Could you check a few things on this model? Use its own coordinates, in mm. Face numbers are marked on the shaded views. A direction names the side the tool comes from. Round coordinates to 2 decimals unless told otherwise and drop trailing zeros. Write each loop counter-clockwise with the first axis right and the second up, starting at its lowest first coordinate (ties: lowest second). Pieces come first, ordered by that corner, then holes. Notation, with made-up numbers: (-16, -35.75) -> (33, -35.75) arc R28 ccw to (33, -9.75) -> close; hole circle Ø10 at (62, 5.25). An arc over 180 degrees is marked (long way). Answer as CSV lines item,"result". Start each with the question number.
Q1. Imagine slicing it at D-D on x = -1.75. Please give me the cut outline in (y, z).
Q2. Imagine slicing it at B-B on x = 0. Please give me the cut outline in (y, z), and give its area (3 significant figures).
Q3. Imagine slicing it at A-A on y = 0. Please give me the cut outline in (x, z), and give its area (3 significant figures).
Q4. For the marked faces 1, 2 and 3, which set-ups out of +Z, -Z, +X, -X, +Y, -Y let a thin tool reach every point of the face, with its end or its side?
Q5. If I drill on line 1 (X direction, y = 0.1, z = 13); line 2 (Z direction, x = 0, y = 0.1); line 3 (Y direction, x = -2, z = 5.25), over which ranges is the centre line in solid material (lowest first)? Write a range as [from, to].
Q6. Will these pins go through, and if not, where does the flat tip stop? pin 1 Ø1 at (x, y) = (3, -1.5) entering from +Z; pin 2 Ø1 at (x, z) = (-3.5, 11) entering from -Y; pin 3 Ø1.1 at (y, z) = (0, 5) entering from -X.
Q7. Imagine slicing it at C-C on z = 13. Please give me the cut outline in (x, y), and give its area (3 significant figures).
Autodesk Inventor part; units mm, degrees
ref_plane "YZ Plane" through (0, 0, 0) normal (1, 0, 0) x (0, 1, 0)
ref_plane "XZ Plane" through (0, 0, 0) normal (0, 1, 0) x (-1, 0, 0)
ref_plane "XY Plane" through (0, 0, 0) normal (0, 0, 1) x (1, 0, 0)
sketch "Skizze1" plane through (0, 0, 0) normal (0, 0, 1) x (1, 0, 0)
  circle A0 centre (0, 0) radius 6.5
  dimension "d11" = 13
extrude "Extrusion1" add sketch "Skizze1" along normal blind 1
sketch "Skizze2" plane through (0, 0, 0) normal (0, 1, 0) x (-1, 0, 0)
  line L0 (6.5, 1) -> (-6.5, 1)
  line L1 (3.5, 1) -> (-3.5, 1)
  line L2 (-3.5, 1) -> (-3.5, 16)
  line L3 (-3.5, 16) -> (3.5, 16)
  line L4 (3.5, 16) -> (3.5, 1)
  line L5 (0, -1) -> (0, 20)
  circle A0 centre (0, 13) radius 1
  line L6 (6.5, 0) -> (-6.5, 0)
  point P0 (-3.5, 1)
  dimension "d2" = 15
  dimension "d3" = 7
  dimension "d4" = 2
  dimension "d5" = 3
  dimension "d12" = 13
extrude "Extrusion2" add sketch "Skizze2" along normal mid plane 1 contours L0 L5 A0 L3 L4 | L0 L2 L3 L5 A0
chamfer "Fase1" distance 2 angle 45 2 edges at (3.5, 0, 16) (-3.5, 0, 16)
properties part number "Deckel"
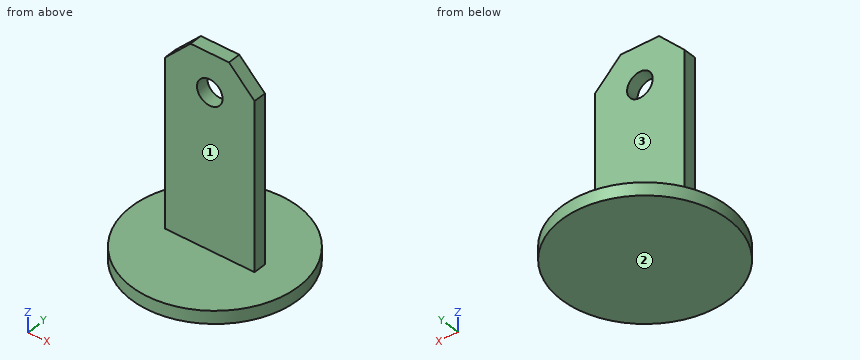
Checks:
1,outline,"(-6.26, 0) -> (6.26, 0) -> (6.26, 1) -> (0.5, 1) -> (0.5, 15.75) -> (-0.5, 15.75) -> (-0.5, 1) -> (-6.26, 1) -> close"
2,outline,"(-6.5, 0) -> (6.5, 0) -> (6.5, 1) -> (0.5, 1) -> (0.5, 12) -> (-0.5, 12) -> (-0.5, 1) -> (-6.5, 1) -> close; (-0.5, 14) -> (0.5, 14) -> (0.5, 16) -> (-0.5, 16) -> close"
2,area,"26.0 mm^2"
3,outline,"(-6.5, 0) -> (6.5, 0) -> (6.5, 1) -> (3.5, 1) -> (3.5, 14) -> (1.5, 16) -> (-1.5, 16) -> (-3.5, 14) -> (-3.5, 1) -> (-6.5, 1) -> close; hole circle Ø2 at (0, 13)"
3,area,"111 mm^2"
4,face 1,"+Z, +X, -X, -Y"
4,face 2,"-Z, +X, -X, +Y, -Y"
4,face 3,"+Z, +X, -X, +Y"
5,line 1,"[-3.5, -1], [1, 3.5]"
5,line 2,"[0, 12], [14, 16]"
5,line 3,"[-0.5, 0.5]"
6,pin 1,"z = 1"
6,pin 2,"y = -0.5"
6,pin 3,"x = -3.5"
7,outline,"(-3.5, -0.5) -> (-1, -0.5) -> (-1, 0.5) -> (-3.5, 0.5) -> close; (1, -0.5) -> (3.5, -0.5) -> (3.5, 0.5) -> (1, 0.5) -> close"
7,area,"5.00 mm^2"
